from build123d import *

# Parameters (mm, degrees)
SKETCH1_W           = 10
SKETCH1_H           = 10
BOSS_EXTRUDE2_DEPTH = 6
CUT_EXTRUDE1_DEPTH  = 3.81
SKETCH3_R           = 31.75
CUT_EXTRUDE2_DEPTH  = 0.3
SKETCH4_R           = 25.019
SKETCH4_W           = 10
SKETCH4_H           = 10
BOSS_EXTRUDE3_DEPTH = 12.065
SKETCH5_R           = 15.875
CUT_EXTRUDE3_DEPTH  = 6.35
FILLET1_R           = 1.3716
CUT_EXTRUDE4_START  = -0.3
SKETCH6_R           = 54.970137174
SKETCH6_R_2         = 31.75
CUT_EXTRUDE4_DEPTH  = 0.3


with BuildPart() as part:
    # Sketch1 → Boss-Extrude2 (new body)
    with BuildSketch(Plane(origin=(0, 0, 0), x_dir=(1, 0, 0), z_dir=(0, 1, 0))):
        with BuildLine():
            Line((35.405449863, 6.5405), (38.565312338, 6.5405))
            ThreePointArc((38.565312338, 6.5405), (27.795594479, 27.522107178), (6.9215, 38.498757042))
            Line((6.9215, 38.498757042), (6.9215, 35.332942957))
            ThreePointArc((6.9215, 35.332942957), (0.19391896, 36.003977776), (-6.5405, 35.405449863))
            Line((-6.5405, 35.405449863), (-6.5405, 38.565312338))
            ThreePointArc((-6.5405, 38.565312338), (-27.522107178, 27.795594479), (-38.498757042, 6.9215))
            Line((-38.498757042, 6.9215), (-35.332942957, 6.9215))
            ThreePointArc((-35.332942957, 6.9215), (-36.003977776, 0.19391896), (-35.405449863, -6.5405))
            Line((-35.405449863, -6.5405), (-38.565312338, -6.5405))
            ThreePointArc((-38.565312338, -6.5405), (-27.795594479, -27.522107178), (-6.9215, -38.498757042))
            Line((-6.9215, -38.498757042), (-6.9215, -35.332942957))
            ThreePointArc((-6.9215, -35.332942957), (-0.19391896, -36.003977776), (6.5405, -35.405449863))
            Line((6.5405, -35.405449863), (6.5405, -38.565312338))
            ThreePointArc((6.5405, -38.565312338), (27.522107178, -27.795594479), (38.498757042, -6.9215))
            Line((38.498757042, -6.9215), (35.332942957, -6.9215))
            ThreePointArc((35.332942957, -6.9215), (36.003977776, -0.19391896), (35.405449863, 6.5405))
        make_face()
        Rectangle(SKETCH1_W, SKETCH1_H, mode=Mode.SUBTRACT)
    extrude(amount=BOSS_EXTRUDE2_DEPTH)

    # Sketch2 → Cut-Extrude1 (cut)
    with BuildSketch(Plane.XZ):
        with BuildLine():
            Line((17.377665752, -10.033), (-0.286554615, -40.628327152))
            ThreePointArc((-0.286554615, -40.628327152), (-2.416432138, -40.557415308), (-4.539661745, -40.374924792))
            Line((-4.539661745, -40.374924792), (8.196212586, -18.315743371))
            ThreePointArc((8.196212586, -18.315743371), (-13.440862054, 14.899247741), (17.377665752, -10.033))
        make_face()
    extrude(amount=-CUT_EXTRUDE1_DEPTH, mode=Mode.SUBTRACT)

    # Sketch3 → Cut-Extrude2 (cut)
    with BuildSketch(Plane.XZ):
        Circle(SKETCH3_R)
    extrude(amount=-CUT_EXTRUDE2_DEPTH, mode=Mode.SUBTRACT)

    # Sketch4 → Boss-Extrude3 (add)
    with BuildSketch(Plane(origin=(0, 6, 0), x_dir=(1, 0, 0), z_dir=(0, 1, 0))):
        with Locations(Location((0, 0, 0), (0, 0, 90))):
            Circle(SKETCH4_R)
        Rectangle(SKETCH4_W, SKETCH4_H, mode=Mode.SUBTRACT)
    extrude(amount=BOSS_EXTRUDE3_DEPTH)

    # Sketch5 → Cut-Extrude3 (cut)
    with BuildSketch(Plane.XZ.offset(-3.81)):
        with Locations(Location((0, 0, 0), (0, 0, 270))):
            Circle(SKETCH5_R)
    extrude(amount=-CUT_EXTRUDE3_DEPTH, mode=Mode.SUBTRACT)

    # Fillet1
    fillet1_edges = [part.edges().sort_by_distance(p)[0] for p in [
        (5, 14.1125, -5),
        (-5, 14.1125, -5),
        (-5, 14.1125, 5),
        (5, 14.1125, 5),
    ]]
    fillet(fillet1_edges, radius=FILLET1_R)

    # Sketch6 → Cut-Extrude4 (cut)
    with BuildSketch(Plane(origin=(0, 6, 0), x_dir=(1, 0, 0), z_dir=(0, 1, 0)).offset(CUT_EXTRUDE4_START)):
        Circle(SKETCH6_R)
        with Locations(Location((0, 0, 0), (0, 0, 270))):
            Circle(SKETCH6_R_2, mode=Mode.SUBTRACT)
    extrude(amount=CUT_EXTRUDE4_DEPTH, mode=Mode.SUBTRACT)


solid = part.part
Input: part model. Units: mm. Frame: model coordinates. A direction names the side the tool comes from. Coordinates: 2 decimals unless noted, no trailing zeros. Loops run counter-clockwise (first coordinate to the right, second up) from the corner with the lowest first, then second, coordinate; pieces in that order, holes last.
(1) Pull-direction query (Z, two-part tool) for faces 4 (the face through (0, 14, 5)), 5 (the face through (-28.031, 2.81, 27.283)), 6 (the face through (6.922, 3, -37)), 7 (the face through (36.003, 2.81, 0.289)); classes: released by +Z, released by -Z, zero draft, split by the parting line, or undercut.
(2) Section A-A on y = 15.75. Return the cut outline in (x, z), then the cut area to 3 significant figures.
(3) Set-up query: faces 1 (the face through (37, 3, 6.922)), 2 (the face through (23.4, 6, -9.6)), 3 (the face through (21, 0.3, 0)). Return all of +Z, -Z, +X, -X, +Y, -Y with unobstructed straight access to the full face (end or side cutting, diameter ignored); none if empty.
(4) Section C-C on z = -26.5. Return the cut outline in (x, y), then the cut area to 3 significant figures.
(5) First-contact query: pin 1 Ø5 at (x, z) = (-26, -27.5) entering from +Y; pin 2 Ø3.5 at (x, y) = (-0.5, 14) entering from -Z; pin 3 Ø6 at (x, y) = (26, 12.5) entering from -Z. Flat tips, straight axial feed; report the tip coordinate or a pass-through.
(6) Material intervals for probe 1 along X at (y, z) = (0.1, 0); probe 2 along X at (y, z) = (7, 0) (3 decimals); probe 3 along Z at (x, y) = (4, 15.25), sorted ascending.
Data:
1. face 4: undercut
1. face 5: released by +Z
1. face 6: zero draft
1. face 7: undercut
2. outline: circle Ø50.04 at (0, 0); hole (-5, -3.63) arc R1.37 ccw to (-3.63, -5) - (3.63, -5) arc R1.37 ccw to (5, -3.63) - (5, 3.63) arc R1.37 ccw to (3.63, 5) - (-3.63, 5) arc R1.37 ccw to (-5, 3.63) - close
2. area: 1,870 mm2
3. face 1: +X, +Y, -Y
3. face 2: +Y
3. face 3: -Y
4. outline: (-28.77, 0) - (-17.49, 0) - (-17.49, 0.3) - (3.47, 0.3) - (3.47, 3.81) - (7.87, 3.81) - (7.87, 0.3) - (17.49, 0.3) - (17.49, 0) - (28.77, 0) - (28.77, 5.7) - (17.49, 5.7) - (17.49, 6) - (-17.49, 6) - (-17.49, 5.7) - (-28.77, 5.7) - close
4. area: 313 mm2
5. pin 1: stops at y = 5.7
5. pin 2: stops at z = -25.02
5. pin 3: stops at z = -9.85
6. probe 1: x = -36 to -31.75, 31.75 to 36
6. probe 2: x = -25.019 to -15.875, 15.875 to 25.019
6. probe 3: z = -24.7 to -4.95, 4.95 to 24.7
